Autodesk Inventor part; units mm, degrees
ref_plane "YZ Plane" through (0, 0, 0) normal (1, 0, 0) x (0, 1, 0)
ref_plane "XZ Plane" through (0, 0, 0) normal (0, 1, 0) x (-1, 0, 0)
ref_plane "XY Plane" through (0, 0, 0) normal (0, 0, 1) x (1, 0, 0)
sketch "Sketch1" plane through (0, 0, 0) normal (0, 0, 1) x (1, 0, 0)
  line L0 (-21.5328, 23.6618) -> (3.4672, 23.6618)
  line L1 (3.4672, 23.6618) -> (3.4672, -1.3382)
  line L2 (3.4672, -1.3382) -> (-21.5328, -1.3382)
  line L3 (-21.5328, -1.3382) -> (-21.5328, 23.6618)
  dimension "d0" = 25
  dimension "d1" = 25
extrude "Extrusion1" add sketch "Sketch1" along normal blind 64
sketch "Sketch2" plane through (0, 0, 64) normal (0, 0, 1) x (1, 0, 0)
  line L0 (3.4672, 23.6618) -> (3.4672, -1.3382)
  line L1 (-21.5328, 23.6618) -> (3.4672, 23.6618)
  line L2 (-21.5328, -1.3382) -> (-21.5328, 23.6618)
  circle A0 centre (-9.0328, 11.1618) radius 12.5 construction
hole "Hole1" at (-9.0328, 11.1618, 64) at (-9.0328, 11.1618, 64) direction (0, 0, -1) diameter 6.35 end through all
properties part number "parameters"
The model under review builds one solid part; all positions refer to its coordinate system, in mm. Give positions to 0.01 mm unless a question says otherwise; leave off trailing zeros. Write each loop counter-clockwise with the first axis right and the second up, starting at its lowest first coordinate (ties: lowest second). Pieces come first, ordered by that corner, then holes. Notation, with made-up numbers: M 27,-14.5 L 81,-14.5 A20 ccw 81,-10.5 Z; hole C 48.25,-33.75 d5. An arc over 180 degrees is marked long. Answer in a Markdown table with one row per item.
Item 1: For line 1 along X through (y, z) = (11, 3); line 2 along Y through (x, z) = (-6.5, 40.5); line 3 along X through (y, z) = (13.5, 36), list the stretches that pass through material, from the lowest coordinate up.
Check sheet entries:
| item | result |
|---|---|
| line 1 | -21.53 to -12.2, -5.86 to 3.47 |
| line 2 | -1.34 to 9.25, 13.08 to 23.66 |
| line 3 | -21.53 to -11.18, -6.88 to 3.47 |
Item 2: Add section B-B on z = 42. Give the boundary of the cut face in (x, y) (3 decimals).
Check sheet entries:
| item | result |
|---|---|
| outline | M -21.533,-1.338 L 3.467,-1.338 L 3.467,23.662 L -21.533,23.662 Z; hole C -9.033,11.162 d6.35 |
Item 3: Draft analysis for pull direction Y (two halves, no side actions). For faces 1 (the face through (-9, 23.662, 32)), 2 (the face through (3.467, 11, 32)), 3 (the face through (-12.18, 11.58, 31.55)), state which applies: +Y half, -Y half, draft (parallel to the pull), parting line (faces both ways), or undercut.
Check sheet entries:
| item | result |
|---|---|
| face 1 | +Y half |
| face 2 | draft |
| face 3 | undercut |
Item 4: For P1, Ø7.5, axis at x = -9.03, y = 11.16, coming from the +Z side, flat-tipped, find the tip position at first contact; note if it passes through.
Check sheet entries:
| item | result |
|---|---|
| P1 | z = 64 |
Item 5: Add section A-A on x = -7.5. Give the boundary of the cut face in (y, z), plus the area to 3 significant figures.
Check sheet entries:
| item | result |
|---|---|
| outline | M -1.34,0 L 8.38,0 L 8.38,64 L -1.34,64 Z; M 13.94,0 L 23.66,0 L 23.66,64 L 13.94,64 Z |
| area | 1,240 mm2 |
